```python
from build123d import *

# Parameters (mm, degrees)
BOSS_EXTRUDE1_DEPTH                                = 50.8
CSK_FOR_10_FLAT_HEAD_MACHINE_SCREW_100_D           = 5.6134
CSK_FOR_10_FLAT_HEAD_MACHINE_SCREW_100_CSINK_D     = 17.78
CSK_FOR_10_FLAT_HEAD_MACHINE_SCREW_100_CSINK_ANGLE = 90
CSK_FOR_10_FLAT_HEAD_MACHINE_SCREW_2_D             = 5.6134
CSK_FOR_10_FLAT_HEAD_MACHINE_SCREW_2_CSINK_D       = 17.78
CSK_FOR_10_FLAT_HEAD_MACHINE_SCREW_2_CSINK_ANGLE   = 90


with BuildPart() as part:
    # Sketch1 → Boss-Extrude1 (new body)
    with BuildSketch(Plane(origin=(0, 0, 0), x_dir=(1, 0, 0), z_dir=(0, 1, 0))):
        Polygon((0, 0), (-50.8, 0), (-50.8, -40.046314449), (0, -46.961736623), align=None)
    extrude(amount=BOSS_EXTRUDE1_DEPTH)

    # CSK for _10 Flat Head Machine Screw _100 (through all)
    with Locations(Plane(origin=(295.341972913, -214.795089466, 50.8), x_dir=(-1, 0, 0), z_dir=(0, 0, 1))):
        with Locations((333.441972913, -227.495089466), (333.441972913, -252.895089466), (333.441972913, -329.095089466), (333.441972913, -354.495089466)):
            CounterSinkHole(CSK_FOR_10_FLAT_HEAD_MACHINE_SCREW_100_D / 2, CSK_FOR_10_FLAT_HEAD_MACHINE_SCREW_100_CSINK_D / 2, counter_sink_angle=CSK_FOR_10_FLAT_HEAD_MACHINE_SCREW_100_CSINK_ANGLE)

    # CSK for _10 Flat Head Machine Screw  2 (through all)
    with Locations(Plane(origin=(295.341972913, -316.395089466, 53.34), x_dir=(-1, 0, 0), z_dir=(0, 0, 1))):
        with Locations((308.041972913, -252.895089466), (308.041972913, -227.495089466), (308.041972913, -329.095089466), (308.041972913, -354.495089466)):
            CounterSinkHole(CSK_FOR_10_FLAT_HEAD_MACHINE_SCREW_2_D / 2, CSK_FOR_10_FLAT_HEAD_MACHINE_SCREW_2_CSINK_D / 2, counter_sink_angle=CSK_FOR_10_FLAT_HEAD_MACHINE_SCREW_2_CSINK_ANGLE)


solid = part.part
```
CAD build for the part. Positions are in the model's coordinates, mm. Give positions to 0.01 mm unless a question says otherwise; leave off trailing zeros. Write each loop counter-clockwise with the first axis right and the second up, starting at its lowest first coordinate (ties: lowest second). Pieces come first, ordered by that corner, then holes. Notation, with made-up numbers: M 27.5,58 L 49.5,58 A21 cw 49.5,89 Z; hole C 86.5,-37 d9. An arc over 180 degrees is marked long. Return JSON: item names as keys, results as strings. Group by question number.
(1) Flat gauge pins, fed straight in: pin 1 Ø9 at (x, y) = (-12.7, 38.1) entering from +Z; pin 2 Ø9 at (x, y) = (-38.1, 12.7) entering from +Z; pin 3 Ø1 at (x, y) = (-6, 27.5) entering from +Z. Where does each tip first touch, or does it go through?
(2) Drill centre lines: L1, parallel to Y at x = -38, z = 20; L2, parallel to X at y = 38, z = 16; L3, parallel to Y at x = -12, z = 26. Where is each one in solid material? Low to high. Write a range as [from, to].
(3) Mould opens along Y. For faces 1 (the face through (-50.8, 25, 20)), 2 (the face through (-26, 50.8, 23)), 3 (the face through (-40.904, 12.577, 20.784)) say: pulls with the +Y half, pulls with the -Y half, needs draft (parallel to the pull), parting line crosses it, or undercut.
(4) Band-saw the part on C-C (x = -11). Give the cut face in (y, z), and give its area (3 significant figures).
(5) Band-saw the part on D-D (y = 28). Give the cut face in (x, z).
(6) Band-saw the part on B-B (z = 33). Give the cut face in (x, y), and give its area (3 significant figures).
(7) Band-saw the part on A-A (y = 38.1). Give the cut face in (x, z), and give its area (3 significant figures).
Entries:
{
 "1": {"pin 1": "stops at z = 45.85", "pin 2": "stops at z = 42.39", "pin 3": "stops at z = 46.21"},
 "2": {"L1": "y = [0, 9.9], [15.5, 35.3], [40.9, 50.8]", "L2": "x = [-50.8, -40.9], [-35.3, -15.5], [-9.9, 0]", "L3": "y = [0, 9.98], [15.42, 35.38], [40.82, 50.8]"},
 "3": {"face 1": "needs draft", "face 2": "pulls with the +Y half", "face 3": "undercut"},
 "4": {"outline": "M 0,0 L 10.47,0 L 10.47,45.46 L 0,45.46 Z; M 14.93,0 L 35.87,0 L 35.87,45.46 L 14.93,45.46 Z; M 40.33,0 L 50.8,0 L 50.8,45.46 L 40.33,45.46 Z", "area": "1,900 mm^2"},
 "5": {"outline": "M -50.8,0 L 0,0 L 0,46.96 L -50.8,40.05 Z"},
 "6": {"outline": "M -50.8,0 L 0,0 L 0,50.8 L -50.8,50.8 Z; hole C -38.1,12.7 d5.61; hole C -38.1,38.1 d5.61; hole C -12.7,12.7 d5.61; hole C -12.7,38.1 d5.61", "area": "2,480 mm^2"},
 "7": {"outline": "M -50.8,0 L -40.91,0 L -40.91,41.39 L -50.8,40.05 Z; M -35.29,0 L -15.51,0 L -15.51,44.85 L -35.29,42.16 Z; M -9.89,0 L 0,0 L 0,46.96 L -9.89,45.61 Z", "area": "1,720 mm^2"}
}
